The listing builds one solid part. Answer for the finished solid, in the listing's coordinates (mm). Face numbers are marked on the shaded views. A direction names the side the tool comes from. Give positions to 0.01 mm unless a question says otherwise; leave off trailing zeros. Write each loop counter-clockwise with the first axis right and the second up, starting at its lowest first coordinate (ties: lowest second). Pieces come first, ordered by that corner, then holes. Notation, with made-up numbers: (63, 13) -> (70, 13) arc R16 cw to (70, 43) -> close; hole circle Ø2 at (24, -30.5). An arc over 180 degrees is marked (long way). Write each question's results on one line, items separated by ' | '. Start each with the question number.
from build123d import *

# Parameters (mm, degrees)
SKETCH_1_R      = 7
EXTRUDE_1_DEPTH = 12
SKETCH_2_R      = 3
EXTRUDE_2_DEPTH = 25
EXTRUDE_3_DEPTH = 6
CHAMFER_1_SIZE  = 0.3


with BuildPart() as part:
    # 草图1 → 凸台-拉伸1 (new body)
    with BuildSketch(Plane.XY):
        Circle(SKETCH_1_R)
    extrude(amount=EXTRUDE_1_DEPTH)

    # 草图2 → 凸台-拉伸2 (add)
    with BuildSketch(Plane.XY.offset(12)):
        Circle(SKETCH_2_R)
    extrude(amount=EXTRUDE_2_DEPTH)

    # 草图3 → 凸台-拉伸3 (add)
    with BuildSketch(Plane.XY.offset(37)):
        Polygon((5, 2.886751346), (0, 5.773502692), (-5, 2.886751346), (-5, -2.886751346), (0, -5.773502692), (5, -2.886751346), align=None)
    extrude(amount=-EXTRUDE_3_DEPTH)

    # 倒角1
    chamfer_1_edges = [part.edges().sort_by_distance(p)[0] for p in [
        (5, 0, 37),
        (2.5, 4.330127019, 37),
        (-2.5, 4.330127019, 37),
        (-5, 0, 37),
        (-2.5, -4.330127019, 37),
        (2.5, -4.330127019, 37),
        (-7, 0, 0),
        (-7, 0, 12),
    ]]
    chamfer(chamfer_1_edges, length=CHAMFER_1_SIZE)


solid = part.part
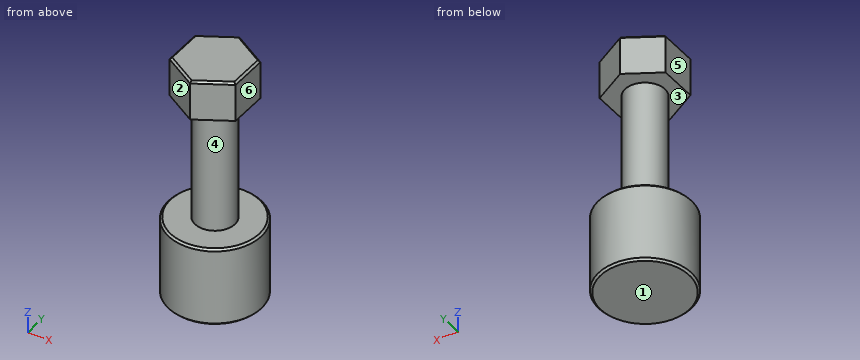
1. Section D-D (z = 3.5) is taken. Write down the section's boundary in (x, y).
2. Section A-A (y = 0) is taken. Write down the section's boundary in (x, z), then the cut area to 3 significant figures.
3. Section B-B (z = 34) is taken. Write down the section's boundary in (x, y).
4. Section C-C (z = 17.5) is taken. Write down the section's boundary in (x, y).
5. Consider probe 1 along Z at (x, y) = (-0.25, 3.25); probe 2 along Z at (x, y) = (-3.75, -5.5); probe 3 along X at (y, z) = (1, 16). Determine where each line is inside the solid, lowest interval first. Write a range as [from, to].
6. The mould has two halves that part along Z. Classify the marked faces 1, 2 and 3: pulls with the +Z half, pulls with the -Z half, needs draft (parallel to the pull), parting line crosses it, or undercut.
7. A tool of negligible diameter and unlimited length cuts with its end or side. For the marked faces 4, 5 and 6, from which of +Z, -Z, +X, -X, +Y, -Y can it reach the whole face along a straight path? Write none if from no direction.
8. Each of these flat-tipped pins is pushed along its axis until it touches: pin 1 Ø6 at (y, z) = (4, 29) entering from +X; pin 2 Ø3 at (x, y) = (-1.5, -0.5) entering from -Z; pin 3 Ø6 at (y, z) = (1, 30) entering from -X; pin 4 Ø5 at (y, z) = (4, 22) entering from -X. Where does it stop, or does it pass through?
Results:
1) outline: circle Ø14 at (0, 0)
2) outline: (-7, 0.3) -> (-6.7, 0) -> (6.7, 0) -> (7, 0.3) -> (7, 11.7) -> (6.7, 12) -> (3, 12) -> (3, 31) -> (5, 31) -> (5, 36.7) -> (4.7, 37) -> (-4.7, 37) -> (-5, 36.7) -> (-5, 31) -> (-3, 31) -> (-3, 12) -> (-6.7, 12) -> (-7, 11.7) -> close | area: 342 mm²
3) outline: (-5, -2.89) -> (0, -5.77) -> (5, -2.89) -> (5, 2.89) -> (0, 5.77) -> (-5, 2.89) -> close
4) outline: circle Ø6 at (0, 0)
5) probe 1: z = [0, 12], [31, 37] | probe 2: z = [0, 12] | probe 3: x = [-2.83, 2.83]
6) face 1: pulls with the -Z half | face 2: needs draft | face 3: undercut
7) face 4: none | face 5: +Z, -X, +Y, -Y | face 6: +Z, +X, +Y, -Y
8) pin 1: stops at x = 5 | pin 2: stops at z = 0 | pin 3: stops at x = -5 | pin 4: stops at x = -2.6
